Build history of the part. All positions in model axes, mm. Face numbers are marked on the shaded views. A direction names the side the tool comes from. Give positions to 0.01 mm unless a question says otherwise; leave off trailing zeros. Loops run counter-clockwise (first coordinate to the right, second up) from the corner with the lowest first, then second, coordinate; pieces in that order, holes last. Notation, with made-up numbers: M 75,-8 L 112,-8 A14 ccw 112,19 Z; hole C -7.5,8 d2. An arc over 180 degrees is marked long. Answer as a JSON object with one key per item and string values. Group by question number.
1. Slice it at A-A (y = -11). List the corners of the cut face in (x, z).
2. Mould opens along Z. For the marked faces 4, 5, 6 and 7 say: released by +Z, released by -Z, zero draft, split by the parting line, or undercut.
3. Slice it at D-D (z = 37). List the corners of the cut face in (x, y).
4. Drill centre lines: line 1 along Y through (x, z) = (57.15, 2) (3 decimals); line 2 along Y through (x, z) = (12.7, 3.5) (3 decimals); line 3 along X through (y, z) = (-8.5, 31.75). Where is each one in solid material? Low to high. Write a range as [from, to].
5. Slice it at C-C (x = 58.5). List the corners of the cut face in (y, z), then the cut area to 3 significant figures.
6. 3-axis set-ups, long thin cutter, end or side, ignore diameter. For the marked faces 1, 2 and 3: which of +Z, -Z, +X, -X, +Y, -Y reach the whole face in a straight line?
7. Drop flat-ended pins along their axis: pin 1 Ø7.5 at (x, z) = (12.7, 31.75) entering from +Y; pin 2 Ø2 at (x, y) = (52.5, -12) entering from +Z; pin 3 Ø6.5 at (y, z) = (-7.5, 26.5) entering from +X. Give the stop position or say it passes through.
8. Slice it at B-B (x = 18). List the corners of the cut face in (y, z).
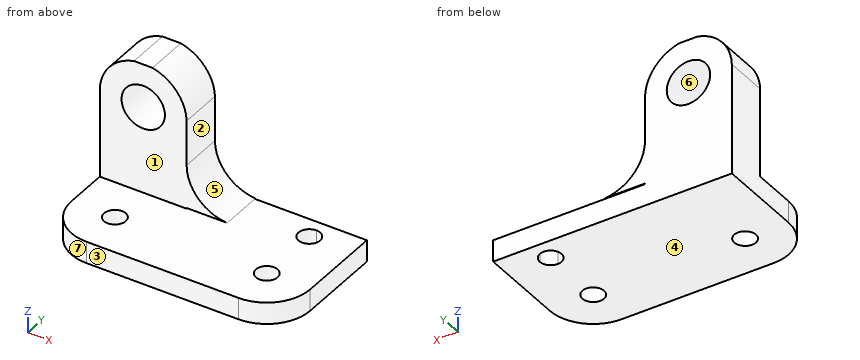
from build123d import *

# Parameters (mm, degrees)
F1_DEPTH  = 38.1
F2_W      = 25.4
F2_H      = 38.1
F3_DEPTH  = 25.4
F4_R      = 6.35
F5_DEPTH  = 12.701
F7_DEPTH  = 12.701
F8_W      = 12.7
F8_H      = 12.7
F9_DEPTH  = 12.7
F11_DEPTH = 12.701
F13_DEPTH = 6.351
F14_R     = 3.175
F15_DEPTH = 6.351


with BuildPart() as f1:
    # F0 (on Front) → F1 (new body)
    with BuildSketch(Plane.XZ):
        Polygon((25.4, 44.45), (0, 44.45), (0, 0), (69.85, 0), (69.85, 6.35), (25.4, 6.35), align=None)
    extrude(amount=F1_DEPTH)

    # F2 (on face) → F3 (cut)
    with BuildSketch(Plane.XZ.offset(38.1)):
        with Locations((12.7, 25.4)):
            Rectangle(F2_W, F2_H)
    extrude(amount=-F3_DEPTH, mode=Mode.SUBTRACT)

    # F4 (on face) → F5 (cut, through all)
    with BuildSketch(Plane.XZ.offset(12.7)):
        with Locations((12.7, 31.75)):
            Circle(F4_R)
    extrude(amount=-F5_DEPTH, mode=Mode.SUBTRACT)

    # F6 (on face) → F7 (cut, through all)
    with BuildSketch(Plane.XZ.offset(12.7)):
        with BuildLine():
            ThreePointArc((0, 32.429072573), (-0.0062022328, 32.0321151685), (0, 31.635157764))
            Line((0, 31.635157764), (0, 32.429072573))
        make_face()
        with BuildLine():
            ThreePointArc((19.05, 31.75), (12.642576534, 38.0997403526), (6.3510385683, 31.635157764))
            Line((6.3510385683, 31.635157764), (19.0489614317, 31.635157764))
            ThreePointArc((19.0489614317, 31.635157764), (19.0497403526, 31.692576534), (19.05, 31.75))
        make_face()
        with BuildLine():
            Line((0, 44.45), (0, 32.429072573))
            ThreePointArc((0, 32.429072573), (2.9352888733, 40.1621823142), (10.0085855964, 44.45))
            Line((10.0085855964, 44.45), (0, 44.45))
        make_face()
        with BuildLine():
            ThreePointArc((15.3914144036, 44.45), (12.7, 44.7383174013), (10.0085855964, 44.45))
            Line((10.0085855964, 44.45), (15.3914144036, 44.45))
        make_face()
        with BuildLine():
            Line((25.4, 32.429072573), (25.4, 31.635157764))
            ThreePointArc((25.4, 31.635157764), (25.4062022328, 32.0321151685), (25.4, 32.429072573))
        make_face()
        with BuildLine():
            Line((25.4, 44.45), (15.3914144036, 44.45))
            ThreePointArc((15.3914144036, 44.45), (22.4647111267, 40.1621823142), (25.4, 32.429072573))
            Line((25.4, 32.429072573), (25.4, 44.45))
        make_face()
    extrude(amount=-F7_DEPTH, mode=Mode.SUBTRACT)

    # F8 (on Front) → F9 (join)
    with BuildSketch(Plane.XZ):
        with Locations((30.9091203046, 12.9094149452)):
            Rectangle(F8_W, F8_H)
    extrude(amount=F9_DEPTH)

    # F10 (on face) → F11 (cut, through all)
    with BuildSketch(Plane.XZ.offset(12.7)):
        with BuildLine():
            Line((37.2591203046, 19.2594149452), (25.4, 19.2594149452))
            ThreePointArc((25.4, 19.2594149452), (28.8257307878, 10.5713666258), (37.2591203046, 6.5594149452))
            Line((37.2591203046, 6.5594149452), (37.2591203046, 19.2594149452))
        make_face()
    extrude(amount=-F11_DEPTH, mode=Mode.SUBTRACT)

    # F12 (on face) → F13 (cut, through all)
    with BuildSketch(Plane.XY.offset(6.35)):
        with BuildLine():
            ThreePointArc((12.7, -38.1), (3.7197438789, -34.3802561211), (0, -25.4))
            Line((0, -25.4), (0, -38.1))
            Line((0, -38.1), (12.7, -38.1))
        make_face()
        with BuildLine():
            ThreePointArc((69.85, -25.4), (66.1302561211, -34.3802561211), (57.15, -38.1))
            Line((57.15, -38.1), (69.85, -38.1))
            Line((69.85, -38.1), (69.85, -25.4))
        make_face()
    extrude(amount=-F13_DEPTH, mode=Mode.SUBTRACT)

    # F14 (on face) → F15 (cut, through all)
    with BuildSketch(Plane.XY.offset(6.35)):
        with BuildLine():
            ThreePointArc((15.875, -25.4), (12.7, -22.225), (9.525, -25.4))
            ThreePointArc((9.525, -25.4), (12.7, -28.575), (15.875, -25.4))
        make_face()
        with Locations((57.15, -25.4)):
            Circle(F14_R)
        with BuildLine():
            Line((57.15, -9.525), (57.15, -3.175))
            ThreePointArc((57.15, -3.175), (53.975, -6.35), (57.15, -9.525))
        make_face()
        with BuildLine():
            ThreePointArc((60.325, -6.35), (59.3950640303, -4.1049359697), (57.15, -3.175))
            Line((57.15, -3.175), (57.15, -9.525))
            ThreePointArc((57.15, -9.525), (59.3950640303, -8.5950640303), (60.325, -6.35))
        make_face()
    extrude(amount=-F15_DEPTH, mode=Mode.SUBTRACT)


solid = f1.part
Established:
{
 "1": {"outline": "M 0,0 L 69.85,0 L 69.85,6.35 L 25.4,6.35 L 25.4,6.56 L 37.26,6.56 A12.73 cw 25.4,19.26 L 25.4,32.43 A12.71 ccw 15.39,44.45 L 10.01,44.45 A12.71 ccw 0,32.43 Z; hole C 12.7,31.75 d12.7"},
 "2": {"face 4": "released by -Z", "face 5": "released by +Z", "face 6": "undercut", "face 7": "zero draft"},
 "3": {"outline": "M 1.01,-12.7 L 9.13,-12.7 L 9.13,0 L 1.01,0 Z; M 16.27,-12.7 L 24.39,-12.7 L 24.39,0 L 16.27,0 Z"},
 "4": {"line 1": "y = [-38.1, -28.575], [-22.225, -9.525], [-3.175, 0]", "line 2": "y = [-38.1, -28.575], [-22.225, 0]", "line 3": "x = [0, 6.35], [19.05, 25.4]"},
 "5": {"outline": "M -38.03,0 L -28.27,0 L -28.27,6.35 L -38.03,6.35 Z; M -22.53,0 L -9.22,0 L -9.22,6.35 L -22.53,6.35 Z; M -3.48,0 L 0,0 L 0,6.35 L -3.48,6.35 Z", "area": "168 mm^2"},
 "6": {"face 1": "+Z, +X, -X, -Y", "face 2": "+Z, +X, +Y, -Y", "face 3": "+Z, -Z, +X, -X, -Y"},
 "7": {"pin 1": "passes through", "pin 2": "stops at z = 6.35", "pin 3": "stops at x = 25.4"},
 "8": {"outline": "M -38.1,0 L 0,0 L 0,28.25 L -12.7,28.25 L -12.7,6.35 L -38.1,6.35 Z; M -12.7,35.25 L 0,35.25 L 0,43.58 L -12.7,43.58 Z"}
}
